The figure shows three views and two pictorial views of one solid part (mm, origin at its lowest corner). Answer the questions. A direction names the side the tool comes from. Round coordinates to 2 decimals unless told otherwise and drop trailing zeros. Order: outer loops, then holes, each group sorted by start corner. A loop starts at its lowest first (then second) coordinate and runs counter-clockwise, first axis right, second up. Notation, with made-up numbers: (-21.75, 36.25) - (-15.75, 36.25) arc R34 cw to (-15.75, 75.25) - close; hole circle Ø4 at (69.25, 39.5). An arc over 180 degrees is marked (long way). Use CSV: the item, a comma, the result in double quotes.
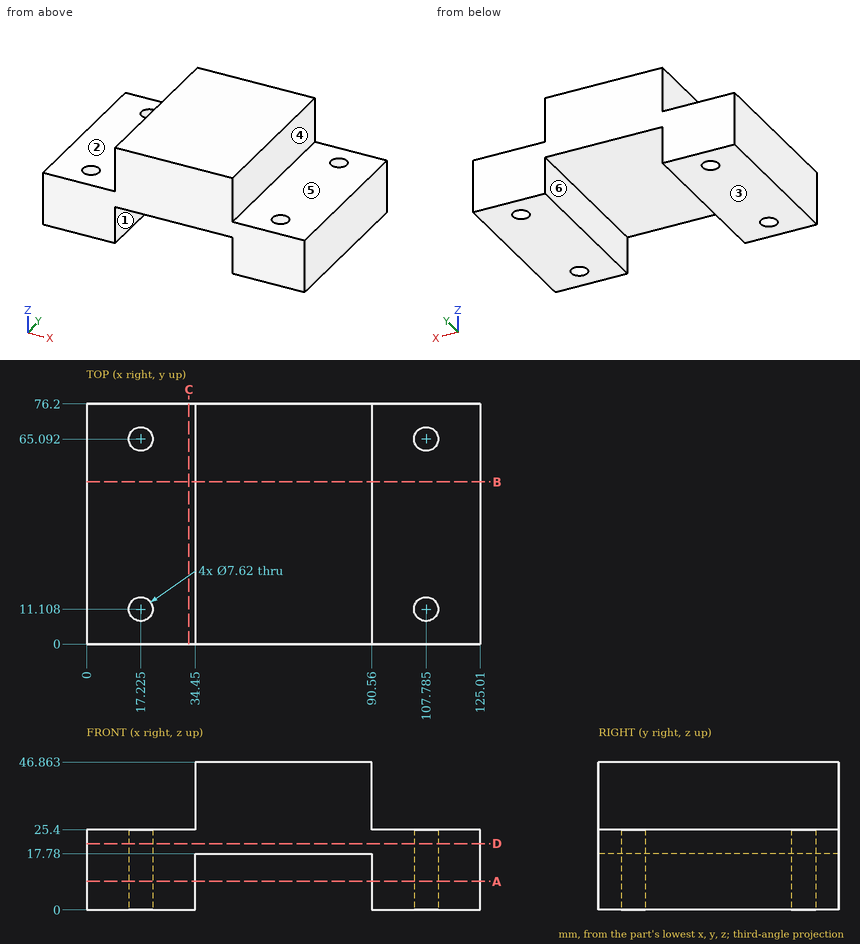
(1) Find section C-C (x = 32.5). Determine the outline of the cut face in (y, z), and give its area (3 significant figures).
Findings below:
outline,"(0, 0) - (76.2, 0) - (76.2, 25.4) - (0, 25.4) - close"
area,"1,940 mm²"
(2) Find section B-B (y = 51.5). Determine the outline of the cut face in (x, z), and give its area (3 significant figures).
Findings below:
outline,"(0, 0) - (34.45, 0) - (34.45, 17.78) - (90.56, 17.78) - (90.56, 0) - (125.01, 0) - (125.01, 25.4) - (90.56, 25.4) - (90.56, 46.86) - (34.45, 46.86) - (34.45, 25.4) - (0, 25.4) - close"
area,"3,380 mm²"
(3) Each of these flat-tipped pins is pushed along its axis until it touches: pin 1 (10.5 mm diameter, centred on y = 44, z = 39.5, fed in from +X); pin 2 (1 mm diameter, centred on y = 31.5, z = 36, fed in from -X); pin 3 (1 mm diameter, centred on x = 72, y = 32, fed in from -Z). Where does it stop, or does it pass through?
Findings below:
pin 1,"stops at x = 90.56"
pin 2,"stops at x = 34.45"
pin 3,"stops at z = 17.78"
(4) The mould has two halves that part along X. Classify the marked faces 4, 5 and 6: released by +X, released by -X, zero draft, split by the parting line, or undercut.
Findings below:
face 4,"released by +X"
face 5,"zero draft"
face 6,"undercut"
(5) Find the intervals of material crossed by L1, parallel to X at y = 57, z = 15; L2, parallel to Y at x = 17.5, z = 18.5; L3, parallel to X at y = 73.5, z = 43, in increasing order. Write a range as from..to.
Findings below:
L1,"x = 0..34.45, 90.56..125.01"
L2,"y = 0..7.31, 14.91..61.29, 68.89..76.2"
L3,"x = 34.45..90.56"
(6) For the marked faces 1, 2 and 3, determine the directions among +Z, -Z, +X, -X, +Y, -Y from which every point of the face is accessible in a straight line to the end or side of a thin tool.
Findings below:
face 1,"-Z, +Y, -Y"
face 2,"+Z, -X, +Y, -Y"
face 3,"-Z, +X, -X, +Y, -Y"
(7) Find section A-A (z = 9). State how many separate pieces and enclosed holes the cut face has, and give its area (3 significant figures).
Findings below:
separate pieces,"2"
enclosed holes,"4"
area,"5,070 mm²"
(8) Find section D-D (z = 21). Determine the outline of the cut face in (x, y) (1 decimal).
Findings below:
outline,"(0, 0) - (125, 0) - (125, 76.2) - (0, 76.2) - close; hole circle Ø7.6 at (17.2, 11.1); hole circle Ø7.6 at (17.2, 65.1); hole circle Ø7.6 at (107.8, 11.1); hole circle Ø7.6 at (107.8, 65.1)"
